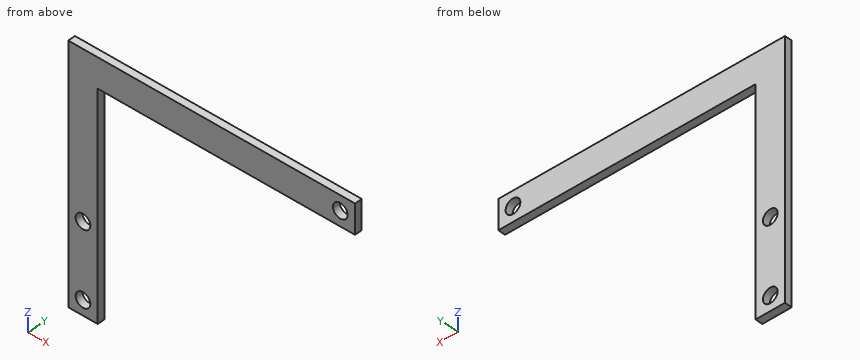
Autodesk Inventor part; units mm, degrees
ref_plane "YZ Plane" through (0, 0, 0) normal (1, 0, 0) x (0, 1, 0)
ref_plane "XZ Plane" through (0, 0, 0) normal (0, 1, 0) x (-1, 0, 0)
ref_plane "XY Plane" through (0, 0, 0) normal (0, 0, 1) x (1, 0, 0)
sketch "スケッチ1" plane through (0, 0, 0) normal (0, 1, 0) x (-1, 0, 0)
  line L0 (234, 0) -> (-39, 0)
  line L1 (0, -204) -> (0, 34)
  line L2 (0, 0) -> (195, 0)
  line L3 (195, 0) -> (195, -170)
  line L4 (175, -20) -> (0, -20)
  circle A0 centre (10, -10) radius 5
  circle A1 centre (185, -110) radius 5
  line L5 (195, -170) -> (175, -170)
  circle A2 centre (185, -160) radius 5
  line L6 (175, -20) -> (175, -170)
  dimension "d0" = 195
  dimension "d2" = 20
  dimension "d3" = 170
  dimension "d5" = 10
  dimension "d6" = 10
  dimension "d7" = 10
  dimension "d8" = 10
  dimension "d9" = 10
  dimension "d23" = 60
  dimension "d24" = 10
  dimension "d30" = 10
  dimension "d31" = 10
  dimension "d34" = 20
extrude "押し出し4" add sketch "スケッチ1" along normal blind 5
properties part number "rocker" material "アルミニウム 6061"
Read the model definition and answer for the solid it produces. Units are mm, in the model's axes. Give positions to 0.01 mm unless a question says otherwise; leave off trailing zeros. Write each loop counter-clockwise with the first axis right and the second up, starting at its lowest first coordinate (ties: lowest second). Pieces come first, ordered by that corner, then holes. Notation, with made-up numbers: (-3.5, -1) -> (15.5, -1) arc R20 ccw to (15.5, 36) -> close; hole circle Ø10 at (-39.75, -18). An arc over 180 degrees is marked (long way). Answer as a JSON object with one key per item and string values.
1) Flat-ended cylindrical pins translate along their axes: pin 1 Ø11.5 at (x, z) = (-10, -10) entering from -Y; pin 2 Ø3 at (y, z) = (2, -110) entering from +X. Find the tip coordinate at first contact, or state that the pin passes through.
Findings below:
{"pin 1": "stops at y = 0", "pin 2": "stops at x = -175"}
2) Section C-C on y = 1 is taken. Write down the section's boundary in (x, z), then the cut area to 3 significant figures.
Findings below:
{"outline": "(-195, -170) -> (-175, -170) -> (-175, -20) -> (0, -20) -> (0, 0) -> (-195, 0) -> close; hole circle Ø10 at (-185, -160); hole circle Ø10 at (-185, -110); hole circle Ø10 at (-10, -10)", "area": "6,660 mm^2"}
3) Section D-D on x = -10 is taken. Write down the section's boundary in (y, z), then the cut area to 3 significant figures.
Findings below:
{"outline": "(0, -20) -> (5, -20) -> (5, -15) -> (0, -15) -> close; (0, -5) -> (5, -5) -> (5, 0) -> (0, 0) -> close", "area": "50.0 mm^2"}
4) Section B-B on x = -185 is taken. Write down the section's boundary in (y, z), then the cut area to 3 significant figures.
Findings below:
{"outline": "(0, -170) -> (5, -170) -> (5, -165) -> (0, -165) -> close; (0, -155) -> (5, -155) -> (5, -115) -> (0, -115) -> close; (0, -105) -> (5, -105) -> (5, 0) -> (0, 0) -> close", "area": "750 mm^2"}
5) Straight lines are drawn through the part: probe 1 along Z at (x, y) = (-185, 1.3); probe 2 along Z at (x, y) = (-10, 4); probe 3 along Z at (x, y) = (-121, 3.05). For each, find the intervals that lie inside material, in ascending order. Write a range as from..to.
Findings below:
{"probe 1": "z = -170..-165, -155..-115, -105..0", "probe 2": "z = -20..-15, -5..0", "probe 3": "z = -20..0"}
6) Section A-A on z = -10 is taken. Write down the section's boundary in (x, y), then the cut area to 3 significant figures.
Findings below:
{"outline": "(-195, 0) -> (-15, 0) -> (-15, 5) -> (-195, 5) -> close; (-5, 0) -> (0, 0) -> (0, 5) -> (-5, 5) -> close", "area": "925 mm^2"}
